```python
from build123d import *

# Parameters (mm, degrees)
F0_R     = 15
F1_DEPTH = 160
F2_W     = 40
F2_H     = 15
F2_W_2   = 18.5
F3_DEPTH = 15
F4_DEPTH = 12.5
F5_DEPTH = 2
F6_DEPTH = 1
F7_DEPTH = 1
F8_W     = 50
F8_H     = 1


with BuildPart() as f1:
    # F0 (on Front) → F1 (new body)
    with BuildSketch(Plane.XZ):
        Circle(F0_R)
    extrude(amount=F1_DEPTH)

    # F2 (on Right) → F3 (cut, symmetric)
    with BuildSketch(Plane.YZ):
        with Locations((-130, -7.5)):
            Rectangle(F2_W, F2_H)
        with Locations((-19.25, -7.5)):
            Rectangle(F2_W_2, F2_H)
    extrude(amount=F3_DEPTH, both=True, mode=Mode.SUBTRACT)

    # F2 (on Right) → F4 (cut, symmetric)
    with BuildSketch(Plane.YZ):
        with Locations((-19.25, -7.5)):
            Rectangle(F2_W_2, F2_H)
        with Locations((-130, -7.5)):
            Rectangle(F2_W, F2_H)
    extrude(amount=F4_DEPTH, both=True, mode=Mode.SUBTRACT)

    # F5 (cut): a face of the model
    f5_faces = [f1.faces().sort_by_distance(p)[0] for p in [
        (0, -110, -6.3661977237),
    ]]
    extrude(f5_faces, amount=-F5_DEPTH, mode=Mode.SUBTRACT)

    # F6 (cut): a face of the model
    f6_faces = [f1.faces().sort_by_distance(p)[0] for p in [
        (0, -28.5, -6.3661977237),
    ]]
    extrude(f6_faces, amount=-F6_DEPTH, mode=Mode.SUBTRACT)

    # F7 (cut): a face of the model
    f7_faces = [f1.faces().sort_by_distance(p)[0] for p in [
        (0, -10, -6.3661977237),
    ]]
    extrude(f7_faces, amount=-F7_DEPTH, mode=Mode.SUBTRACT)

    # F8 (on Right) → F9 (revolve, cut)
    with BuildSketch(Plane.YZ):
        with Locations((-67.068171382, 14.5)):
            Rectangle(F8_W, F8_H)
    revolve(axis=Axis((0, -80.4968252778, 0), (0, -1, 0)), mode=Mode.SUBTRACT)


solid = f1.part
```
For this review, take the finished solid that the model builds, in its own axes (mm). A direction names the side the tool comes from. Coordinates: 2 decimals unless noted, no trailing zeros. Loops run counter-clockwise (first coordinate to the right, second up) from the corner with the lowest first, then second, coordinate; pieces in that order, holes last.
1. For faces 1 (the cylindrical face through (-1.953, -20.74, 14.872)), 2 (the cylindrical face through (5.362, -66.718, 12.932)), 3 (the flat face through (0, -129, 0)), list the 3-axis set-ups (+Z, -Z, +X, -X, +Y, -Y) from which the entire face can be reached by the end or side of a thin tool; tool diameter is ignored.
2. Add section C-C, the plane y = -127.5. Give the boundary of the cut face in (x, z).
3. Insertion check: P1, Ø4, axis at x = 8.5, y = -37.5, coming from the +Z side; P2, Ø9, axis at x = -1, y = -123.5, coming from the -Z side; P3, Ø2, axis at x = 5, y = -97, coming from the +Z side. Each pin has a flat end and moves straight along its axis. Give the tip position at first contact, or say it passes through.
4. Mouldability with a two-part tool opening along Y and no side actions: class faces 4 (the flat face through (0, -160, 0)), 5 (the flat face through (0, 0, 0)), 6 (the flat face through (0, -9, -6)) as +Y half, -Y half, draft (parallel to the pull), parting line (faces both ways), or undercut.
5. Add section D-D, the plane x = -7.5. Give the boundary of the cut face in (y, z), then the cut area to 3 significant figures.
6. Add section A-A, the plane x = 0. Give the boundary of the cut face in (y, z).
7. Add section B-B, the plane z = 3.75. Give the boundary of the cut face in (x, y).
8. For line 1 (Y direction, x = 3, z = -1.25); line 2 (Y direction, x = -10.25, z = 10); line 3 (Z direction, x = 0.5, y = -117), list the stretches that pass through material, from the lowest coordinate up.
Result:
1. face 1: +Y, -Y
1. face 2: none
1. face 3: -Z, +X, -X
2. outline: (-15, 0) - (15, 0) arc R15 ccw to start
3. P1: stops at z = 13.52
3. P2: stops at z = 0
3. P3: stops at z = 14.46
4. face 4: -Y half
4. face 5: +Y half
4. face 6: undercut
5. outline: (-160, -12.99) - (-150, -12.99) - (-150, 0) - (-108, 0) - (-108, -12.99) - (-92.07, -12.99) - (-92.07, -11.82) - (-42.07, -11.82) - (-42.07, -12.99) - (-29.5, -12.99) - (-29.5, 0) - (-9, 0) - (-9, -12.99) - (0, -12.99) - (0, 12.99) - (-42.07, 12.99) - (-42.07, 11.82) - (-92.07, 11.82) - (-92.07, 12.99) - (-160, 12.99) - close
5. area: 3,230 mm2
6. outline: (-160, -15) - (-150, -15) - (-150, 0) - (-108, 0) - (-108, -15) - (-92.07, -15) - (-92.07, -14) - (-42.07, -14) - (-42.07, -15) - (-29.5, -15) - (-29.5, 0) - (-9, 0) - (-9, -15) - (0, -15) - (0, 15) - (-42.07, 15) - (-42.07, 14) - (-92.07, 14) - (-92.07, 15) - (-160, 15) - close
7. outline: (-14.52, -160) - (14.52, -160) - (14.52, -92.07) - (13.49, -92.07) - (13.49, -42.07) - (14.52, -42.07) - (14.52, 0) - (-14.52, 0) - (-14.52, -42.07) - (-13.49, -42.07) - (-13.49, -92.07) - (-14.52, -92.07) - close
8. line 1: y = -160 to -150, -108 to -29.5, -9 to 0
8. line 2: y = -160 to -92.07, -42.07 to 0
8. line 3: z = 0 to 14.99
